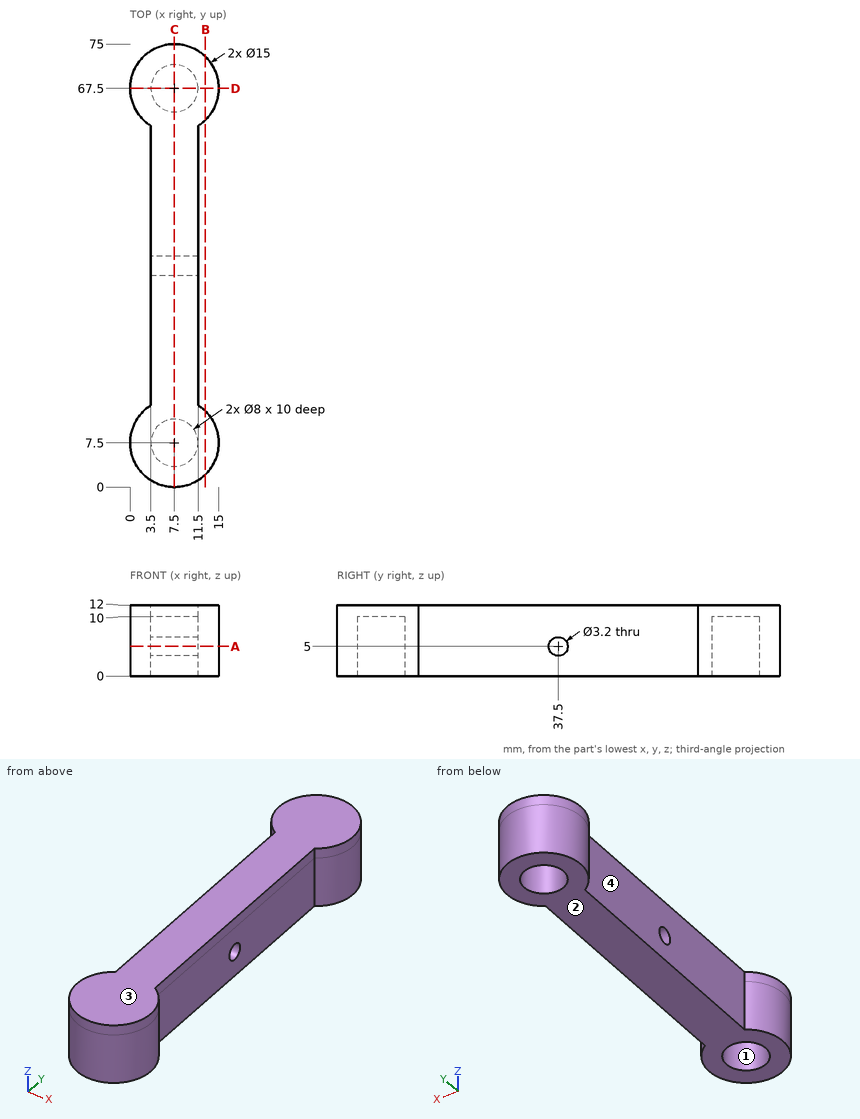
Geometry: see drawing. Coordinates: mm, zero at the bounding-box minimum. A direction names the side the tool comes from. Round coordinates to 2 decimals unless told otherwise and drop trailing zeros. Loops run counter-clockwise (first coordinate to the right, second up) from the corner with the lowest first, then second, coordinate; pieces in that order, holes last.
(1) Material intervals for probe 1 along Y at (x, z) = (7.5, 8); probe 2 along Y at (x, z) = (4, 0.75); probe 3 along Y at (x, z) = (7.5, 5.25), sorted ascending.
From the geometry:
probe 1: y = 0 to 3.5, 11.5 to 63.5, 71.5 to 75
probe 2: y = 0.87 to 5.56, 9.44 to 65.56, 69.44 to 74.13
probe 3: y = 0 to 3.5, 11.5 to 35.92, 39.08 to 63.5, 71.5 to 75
(2) Pull-direction query (Y, two-part tool) for the marked faces 3 and 4; classes: +Y half, -Y half, draft (parallel to the pull), parting line (faces both ways), or undercut.
From the geometry:
face 3: draft
face 4: undercut
(3) Section query A-A (z = 5). Output: boundary loops of the cut face in (x, y).
From the geometry:
outline: (3.5, 13.84) arc R7.5 ccw (long way) to (11.5, 13.84) - (11.5, 35.9) - (3.5, 35.9) - close; (3.5, 39.1) - (11.5, 39.1) - (11.5, 61.16) arc R7.5 ccw (long way) to (3.5, 61.16) - close; hole circle Ø8 at (7.5, 7.5); hole circle Ø8 at (7.5, 67.5)
(4) Section query D-D (y = 67.5). Output: boundary loops of the cut face in (x, z), and give its area (4 significant figures).
From the geometry:
outline: (0, 0) - (3.5, 0) - (3.5, 10) - (11.5, 10) - (11.5, 0) - (15, 0) - (15, 12) - (0, 12) - close
area: 100.0 mm2
(5) Access query for the marked faces 1 and 2. Directions: +Z, -Z, +X, -X, +Y, -Y. A direction counts if a zero-diameter tool reaches every point of the face in a straight line with its end or side. Return the directions, or none.
From the geometry:
face 1: -Z
face 2: -Z, +X, -X, +Y, -Y
(6) Section query B-B (x = 12.75). Output: boundary loops of the cut face in (y, z).
From the geometry:
outline: (2.14, 0) - (12.86, 0) - (12.86, 12) - (2.14, 12) - close; (62.14, 0) - (72.86, 0) - (72.86, 12) - (62.14, 12) - close
(7) Contact query for flat-ended pins moving along their axis: pin 1 Ø1.5 at (x, y) = (12.5, 19) entering from -Z; pin 2 Ø1.5 at (x, z) = (4.5, 5) entering from +Y; pin 3 Ø6 at (y, z) = (43, 6.5) entering from -X; pin 4 Ø7 at (x, y) = (7.5, 67.5) entering from -Z. Output: stop coordinate, or through.
From the geometry:
pin 1: passes through
pin 2: stops at y = 74.65
pin 3: stops at x = 3.5
pin 4: stops at z = 10
(8) Section query C-C (x = 7.5). Output: boundary loops of the cut face in (y, z), and give its area (3 significant figures).
From the geometry:
outline: (0, 0) - (3.5, 0) - (3.5, 10) - (11.5, 10) - (11.5, 0) - (63.5, 0) - (63.5, 10) - (71.5, 10) - (71.5, 0) - (75, 0) - (75, 12) - (0, 12) - close; hole circle Ø3.2 at (37.5, 5)
area: 732 mm2
